Geometry: final body of the model. Coordinates: model frame, mm. A direction names the side the tool comes from. Coordinates: 2 decimals unless noted, no trailing zeros. Write each loop counter-clockwise with the first axis right and the second up, starting at its lowest first coordinate (ties: lowest second). Pieces come first, ordered by that corner, then holes.
from build123d import *

# Parameters (mm, degrees)
MODEL_R             = 3.25
BOSS_EXTRUDE1_DEPTH = 6.6


with BuildPart() as part:
    # Model → Boss-Extrude1 (new body)
    with BuildSketch(Plane.XY):
        with BuildLine():
            Line((58.01, 31.9), (50.31, 31.9))
            ThreePointArc((50.31, 31.9), (48.542233047, 31.167766953), (47.81, 29.4))
            Line((47.81, 29.4), (47.81, 25.4))
            Line((47.81, 25.4), (2.5, 25.4))
            ThreePointArc((2.5, 25.4), (0.732233047, 24.667766953), (0, 22.9))
            Line((0, 22.9), (0, 2.5))
            ThreePointArc((0, 2.5), (0.732233047, 0.732233047), (2.5, 0))
            Line((2.5, 0), (47.81, 0))
            Line((47.81, 0), (47.81, -4))
            ThreePointArc((47.81, -4), (48.542233047, -5.767766953), (50.31, -6.5))
            Line((50.31, -6.5), (58.01, -6.5))
            ThreePointArc((58.01, -6.5), (59.777766953, -5.767766953), (60.51, -4))
            Line((60.51, -4), (60.51, 29.4))
            ThreePointArc((60.51, 29.4), (59.777766953, 31.167766953), (58.01, 31.9))
        make_face()
        with Locations((12.264807358, 12.7)):
            Circle(MODEL_R, mode=Mode.SUBTRACT)
    extrude(amount=BOSS_EXTRUDE1_DEPTH)


solid = part.part
Item 1: Pull-direction query (Y, two-part tool) for faces 1 (the flat face through (47.81, -2, 3)), 2 (the cylindrical face through (13.764, 9.817, 3.254)), 3 (the cylindrical face through (59.797, 31.148, 3.254)); classes: released by +Y, released by -Y, zero draft, split by the parting line, or undercut.
Derived:
face 1: zero draft
face 2: undercut
face 3: released by +Y
Item 2: Section D-D, the plane x = 48.5. Output: boundary loops of the cut face in (y, z).
Derived:
outline: (-5.72, 0) - (31.12, 0) - (31.12, 6.6) - (-5.72, 6.6) - close
Item 3: Section A-A, the plane y = 12.7. Output: boundary loops of the cut face in (x, z), plus the area to 3 significant figures.
Derived:
outline: (0, 0) - (9.01, 0) - (9.01, 6.6) - (0, 6.6) - close; (15.51, 0) - (60.51, 0) - (60.51, 6.6) - (15.51, 6.6) - close
area: 356 mm2
Item 4: Set-up query: faces 4 (the flat face through (47.81, 27, 3)), 5 (the flat face through (25, 0, 3)), 6 (the flat face through (54, 31.9, 3)). Return all of +Z, -Z, +X, -X, +Y, -Y with unobstructed straight access to the full face (end or side cutting, diameter ignored); none if empty.
Derived:
face 4: +Z, -Z, -X, +Y
face 5: +Z, -Z, -X, -Y
face 6: +Z, -Z, +X, -X, +Y
Item 5: Section C-C, the plane x = 17. Output: boundary loops of the cut face in (y, z).
Derived:
outline: (0, 0) - (25.4, 0) - (25.4, 6.6) - (0, 6.6) - close
Item 6: Pin query (flat end, axial travel): pin 1 (1.2 mm diameter, centred on y = -2, z = 3, fed in from -X); pin 2 (3.5 mm diameter, centred on x = 16, z = 4.5, fed in from -Y). Return the tip coordinate at first contact, or that it passes through.
Derived:
pin 1: stops at x = 47.81
pin 2: stops at y = 0
Item 7: Material intervals for probe 1 along Y at (x, z) = (39.5, 4.75); probe 2 along X at (y, z) = (15, 3.5); probe 3 along X at (y, z) = (-2, 3), sorted ascending.
Derived:
probe 1: y = 0 to 25.4
probe 2: x = 0 to 9.97, 14.56 to 60.51
probe 3: x = 47.81 to 60.51
Item 8: Section B-B, the plane z = 5.5. Output: boundary loops of the cut face in (x, y).
Derived:
outline: (0, 2.5) arc R2.5 ccw to (2.5, 0) - (47.81, 0) - (47.81, -4) arc R2.5 ccw to (50.31, -6.5) - (58.01, -6.5) arc R2.5 ccw to (60.51, -4) - (60.51, 29.4) arc R2.5 ccw to (58.01, 31.9) - (50.31, 31.9) arc R2.5 ccw to (47.81, 29.4) - (47.81, 25.4) - (2.5, 25.4) arc R2.5 ccw to (0, 22.9) - close; hole circle Ø6.5 at (12.26, 12.7)
